Work out the finished part from the listing and answer in its coordinate system (mm). A direction names the side the tool comes from. Round coordinates to 2 decimals unless told otherwise and drop trailing zeros. Write each loop counter-clockwise with the first axis right and the second up, starting at its lowest first coordinate (ties: lowest second). Pieces come first, ordered by that corner, then holes.
from build123d import *

# Parameters (mm, degrees)
F0_R     = 14.796322
F1_DEPTH = 6.35


with BuildPart() as f1:
    # F0 (on Top) → F1 (new body)
    with BuildSketch(Plane.XY):
        with BuildLine():
            Line((-27.206885, 22.783245), (-23.203398, 22.783245))
            ThreePointArc((-23.203398, 22.783245), (-119.245242, -4.061273), (-20.152583, -15.255412))
            Line((-20.152583, -15.255412), (-27.206885, -15.255412))
            Line((-27.206885, -15.255412), (-27.206885, 22.783245))
        make_face()
        with Locations((-90.329006, 0)):
            Circle(F0_R, mode=Mode.SUBTRACT)
        with BuildLine():
            ThreePointArc((-23.203398, 22.783245), (-19.175133, 11.70671), (-17.807844, 0))
            ThreePointArc((-17.807844, 0), (-18.397451, -7.717276), (-20.152583, -15.255412))
            Line((-20.152583, -15.255412), (88.56295, -15.255412))
            Line((88.56295, -15.255412), (103.171997, 0))
            Line((103.171997, 0), (88.56295, 22.783245))
            Line((88.56295, 22.783245), (78.915462, 22.783245))
            Line((78.915462, 22.783245), (72.024398, 12.584476))
            Line((72.024398, 12.584476), (59.896126, 12.584476))
            Line((59.896126, 12.584476), (55.534395, 19.386727))
            Line((55.534395, 19.386727), (43.63323, 19.386727))
            Line((43.63323, 19.386727), (36.742169, 12.584476))
            Line((36.742169, 12.584476), (26.543396, 12.584476))
            Line((26.543396, 12.584476), (22.181664, 19.386727))
            Line((22.181664, 19.386727), (8.075351, 19.386727))
            Line((8.075351, 19.386727), (4.758361, 14.796322))
            Line((4.758361, 14.796322), (-7.360628, 14.796322))
            Line((-7.360628, 14.796322), (-7.360628, 22.783245))
            Line((-7.360628, 22.783245), (-23.203398, 22.783245))
        make_face()
        with BuildLine():
            ThreePointArc((-20.152583, -15.255412), (-18.397451, -7.717276), (-17.807844, 0))
            ThreePointArc((-17.807844, 0), (-19.175133, 11.70671), (-23.203398, 22.783245))
            Line((-23.203398, 22.783245), (-27.206885, 22.783245))
            Line((-27.206885, 22.783245), (-27.206885, -15.255412))
            Line((-27.206885, -15.255412), (-20.152583, -15.255412))
        make_face()
    extrude(amount=F1_DEPTH)


solid = f1.part
Q1. Find section B-B (x = 57.5). Determine the outline of the cut face in (y, z).
Q2. Find section A-A (y = -9). Determine the outline of the cut face in (x, z).
Q3. Given pin 1 (1.5 mm diameter, centred on y = 40.5, z = 2.5, fed in from -X); pin 2 (1.9 mm diameter, centred on x = 84, z = 2.5, fed in from +Y); pin 3 (3 mm diameter, centred on y = 21.5, z = 1, fed in from +X); pin 4 (23.5 mm diameter, centred on x = -90.33, y = 0, fed in from -Z), each flat-ended and moving along its own axis, determine where each tip first touches the part or whether it passes through.
Q4. Find the intervals of material crossed by L1, parallel to Y at x = -13, z = 5.5; L2, parallel to Y at x = 72, z = 2.75; L3, parallel to X at y = -3.5, z = 4.25, in increasing order.
Q5. The mould has two halves that part along X. Classify faces 5 (the face through (75.52, 17.76, 3.13)), 6 (the face through (95.8, -7.7, 3.1)), 7 (the face through (40.2, 16, 3.1)), 8 (the face through (-34, 1, 6.35)): +X half, -X half, draft (parallel to the pull), parting line (faces both ways), or undercut.
Q6. A tool of negligible diameter and unlimited length cuts with its end or side. For faces 1 (the face through (33, -15.255, 3)), 2 (the face through (-119.364, -2.105, 3.131)), 3 (the face through (15, 19.387, 3)), 4 (the face through (84, 22.783, 3)), from which of +Z, -Z, +X, -X, +Y, -Y can it reach the whole face along a straight path? Write none if from no direction.
Q7. Find section C-C (y = -33). Determine the outline of the cut face in (x, z).
Report:
1. outline: (-15.26, 0) - (16.32, 0) - (16.32, 6.35) - (-15.26, 6.35) - close
2. outline: (-118.6, 0) - (-102.07, 0) - (-102.07, 6.35) - (-118.6, 6.35) - close; (-78.58, 0) - (94.55, 0) - (94.55, 6.35) - (-78.58, 6.35) - close
3. pin 1: stops at x = -100.24
3. pin 2: stops at y = 22.78
3. pin 3: stops at x = 90.35
3. pin 4: passes through
4. L1: y = -15.26 to 22.78
4. L2: y = -15.26 to 12.58
4. L3: x = -119.29 to -104.71, -75.95 to 99.82
5. face 5: undercut
5. face 6: +X half
5. face 7: undercut
5. face 8: draft
6. face 1: +Z, -Z, +X, -Y
6. face 2: +Z, -Z
6. face 3: +Z, -Z, +Y
6. face 4: +Z, -Z, +X, +Y
7. outline: (-107.23, 0) - (-29.99, 0) - (-29.99, 6.35) - (-107.23, 6.35) - close
